Can you work these out from the drawing? Everything is in mm from the part's minimum corner. A direction names the side the tool comes from. Coordinates: 2 decimals unless noted, no trailing zeros. Order: outer loops, then holes, each group sorted by start corner. A loop starts at its lowest first (then second) coordinate and runs counter-clockwise, first axis right, second up. Notation, with made-up numbers: M -31.75,-2 L -12.75,-2 A11 cw -12.75,7 Z; hole C 21,16.5 d3. An arc over 180 degrees is marked long. Answer as a JSON object with one key per item and string values.
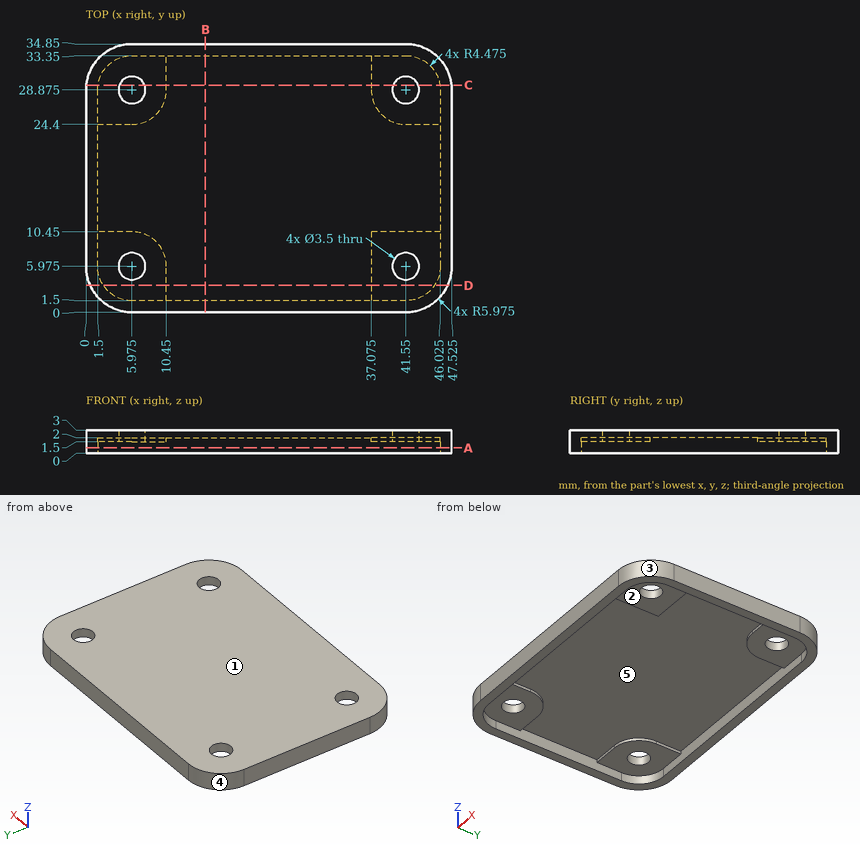
Item 1: I want a section at D-D, the plane y = 3.5. Write out the boundary of the cut face in (x, z) (3 decimals), plus the area to 3 significant figures.
Answers follow:
{"outline": "M 0.537,0 L 2.247,0 L 2.247,1.5 L 10.45,1.5 L 10.45,2 L 37.075,2 L 37.075,1.5 L 45.278,1.5 L 45.278,0 L 46.988,0 L 46.988,3 L 0.537,3 Z", "area": "61.5 mm^2"}
Item 2: I want a section at A-A, the plane z = 0.7. Write out the boundary of the cut face in (x, y) (3 decimals), plus the area to 3 significant figures.
Answers follow:
{"outline": "M 0,5.975 A5.975 ccw 5.975,0 L 41.55,0 A5.975 ccw 47.525,5.975 L 47.525,28.875 A5.975 ccw 41.55,34.85 L 5.975,34.85 A5.975 ccw 0,28.875 Z; hole M 1.5,5.975 A4.475 ccw 5.975,1.5 L 41.55,1.5 A4.475 ccw 46.025,5.975 L 46.025,28.875 A4.475 ccw 41.55,33.35 L 5.975,33.35 A4.475 ccw 1.5,28.875 Z", "area": "225 mm^2"}
Item 3: Please list where these lines run through material, in increasing order: line 1 (Y direction, x = 41.55, z = 1.95) (3 decimals); line 2 (X direction, y = 7, z = 0.9) (3 decimals); line 3 (Y direction, x = 21.5, z = 1.65).
Answers follow:
{"line 1": "y = 0 to 4.225, 7.725 to 10.45, 24.4 to 27.125, 30.625 to 34.85", "line 2": "x = 0 to 1.5, 46.025 to 47.525", "line 3": "y = 0 to 1.5, 33.35 to 34.85"}
Item 4: Which directions (+Z, -Z, +X, -X, +Y, -Y) give clear straight access to the entire face, cutting with the end or side of a thin tool? Please do the marked faces 4 and 5.
Answers follow:
{"face 4": "+Z, -Z, -X, +Y", "face 5": "-Z"}
Item 5: I'm going to push flat-ended pins straight in: pin 1 (0.6 mm diameter, centred on x = 4, z = 2, fed in from +Y); pin 2 (0.6 mm diameter, centred on x = 28.5, z = 1, fed in from -Y); pin 3 (3 mm diameter, centred on x = 41.55, y = 28.875, fed in from +Z); pin 4 (7 mm diameter, centred on x = 40.5, y = 29.5, fed in from -Z). Where does each tip first touch, or does it pass through?
Answers follow:
{"pin 1": "stops at y = 34.61", "pin 2": "stops at y = 0", "pin 3": "passes through", "pin 4": "stops at z = 1.5"}
Item 6: I want a section at C-C, the plane y = 29.5. Write out the boundary of the cut face in (x, z) (3 decimals).
Answers follow:
{"outline": "M 0.033,0 L 1.544,0 L 1.544,1.5 L 4.34,1.5 L 4.34,3 L 0.033,3 Z; M 7.61,1.5 L 10.45,1.5 L 10.45,2 L 37.075,2 L 37.075,1.5 L 39.915,1.5 L 39.915,3 L 7.61,3 Z; M 43.185,1.5 L 45.981,1.5 L 45.981,0 L 47.492,0 L 47.492,3 L 43.185,3 Z"}
Item 7: If we mould it in two halves opening along Y, with no side actions, what happens to the marked faces 1, 2 and 3? For each: pulls with the +Y half, pulls with the -Y half, needs draft (parallel to the pull), parting line crosses it, or undercut.
Answers follow:
{"face 1": "needs draft", "face 2": "undercut", "face 3": "pulls with the -Y half"}
Item 8: I want a section at B-B, the plane x = 15.5. Write out the boundary of the cut face in (y, z), plus the area to 4 significant figures.
Answers follow:
{"outline": "M 0,0 L 1.5,0 L 1.5,2 L 33.35,2 L 33.35,0 L 34.85,0 L 34.85,3 L 0,3 Z", "area": "40.85 mm^2"}
